from build123d import *

# Parameters (mm, degrees)
SKETCH_1_W          = 18.4
SKETCH_1_H          = 7
EXTRUDE_1_DEPTH     = 9.8
SKETCH_2_R          = 1.6
CUT_EXTRUDE_1_DEPTH = 9.8
FILLET_1_R          = 0.5


with BuildPart() as part:
    # 草图1 → 凸台-拉伸1 (new body)
    with BuildSketch(Plane.XY):
        with Locations((9.2, 3.5)):
            Rectangle(SKETCH_1_W, SKETCH_1_H)
    extrude(amount=EXTRUDE_1_DEPTH)

    # 草图2 → 切除-拉伸1 (cut)
    with BuildSketch(Plane.XY.offset(9.8)):
        with Locations((4.3, 3.5)):
            Circle(SKETCH_2_R)
        with Locations((14.1, 3.5)):
            Circle(SKETCH_2_R)
    extrude(amount=-CUT_EXTRUDE_1_DEPTH, mode=Mode.SUBTRACT)

    # 圆角1
    fillet_1_edges = [part.edges().sort_by_distance(p)[0] for p in [
        (18.4, 3.5, 9.8),
        (9.2, 7, 9.8),
        (0, 3.5, 9.8),
        (9.2, 7, 0),
        (18.4, 3.5, 0),
        (9.2, 0, 0),
        (0, 3.5, 0),
        (0, 7, 4.9),
        (18.4, 7, 4.9),
        (18.4, 0, 4.9),
        (0, 0, 4.9),
        (9.2, 0, 9.8),
    ]]
    fillet(fillet_1_edges, radius=FILLET_1_R)


solid = part.part
Geometry check sheet. Reference: the model listing, model coordinates, mm. Round coordinates to 2 decimals unless told otherwise and drop trailing zeros. Order: outer loops, then holes, each group sorted by start corner. A loop starts at its lowest first (then second) coordinate and runs counter-clockwise, first axis right, second up. Notation, with made-up numbers: (41.5, 34) - (79.5, 34) arc R19 cw to (79.5, 61) - close; hole circle Ø7 at (9.25, 24.25). An arc over 180 degrees is marked (long way). One line per question, with ' | ' between items. Start each with the question number.
(1) Sectioned sample at B-B on x = 4.3. Record the cut outline in (y, z), and give its area (3 significant figures).
(2) Thickness scan on L1, parallel to Y at x = 4.3, z = 5.25; L2, parallel to X at y = 3.75, z = 0.5; L3, parallel to X at y = 4.75, z = 7.25. Record the ranges inside material, lowest first. Write a range as [from, to].
(3) Release check for a two-part mould opening along X. For faces 1 (the flat face through (0, 3, 5)), 2 (the cylindrical face through (5.826, 3.981, 4.969)), 3 (the cylindrical face through (15.626, 3.981, 4.969)), 4 (the flat face through (9, 7, 5)) record: released by +X, released by -X, zero draft, split by the parting line, or undercut.
(4) Sectioned sample at C-C on z = 7.25. Record the cut outline in (x, y).
(5) Sectioned sample at D-D on y = 2.5. Record the cut outline in (x, z).
(6) Sectioned sample at A-A on y = 3.5. Record the cut outline in (x, z), and give its area (3 significant figures).
Conclusion:
1) outline: (0, 0.5) arc R0.5 ccw to (0.5, 0) - (1.9, 0) - (1.9, 9.8) - (0.5, 9.8) arc R0.5 ccw to (0, 9.3) - close; (5.1, 0) - (6.5, 0) arc R0.5 ccw to (7, 0.5) - (7, 9.3) arc R0.5 ccw to (6.5, 9.8) - (5.1, 9.8) - close | area: 37.0 mm2
2) L1: y = [0, 1.9], [5.1, 7] | L2: x = [0, 2.72], [5.88, 12.52], [15.68, 18.4] | L3: x = [0, 3.3], [5.3, 13.1], [15.1, 18.4]
3) face 1: released by -X | face 2: undercut | face 3: undercut | face 4: zero draft
4) outline: (0, 0.5) arc R0.5 ccw to (0.5, 0) - (17.9, 0) arc R0.5 ccw to (18.4, 0.5) - (18.4, 6.5) arc R0.5 ccw to (17.9, 7) - (0.5, 7) arc R0.5 ccw to (0, 6.5) - close; hole circle Ø3.2 at (4.3, 3.5); hole circle Ø3.2 at (14.1, 3.5)
5) outline: (0, 0.5) arc R0.5 ccw to (0.5, 0) - (3.05, 0) - (3.05, 9.8) - (0.5, 9.8) arc R0.5 ccw to (0, 9.3) - close; (5.55, 0) - (12.85, 0) - (12.85, 9.8) - (5.55, 9.8) - close; (15.35, 0) - (17.9, 0) arc R0.5 ccw to (18.4, 0.5) - (18.4, 9.3) arc R0.5 ccw to (17.9, 9.8) - (15.35, 9.8) - close
6) outline: (0, 0.5) arc R0.5 ccw to (0.5, 0) - (2.7, 0) - (2.7, 9.8) - (0.5, 9.8) arc R0.5 ccw to (0, 9.3) - close; (5.9, 0) - (12.5, 0) - (12.5, 9.8) - (5.9, 9.8) - close; (15.7, 0) - (17.9, 0) arc R0.5 ccw to (18.4, 0.5) - (18.4, 9.3) arc R0.5 ccw to (17.9, 9.8) - (15.7, 9.8) - close | area: 117 mm2
